For this review, take the finished solid that the model builds, in its own axes (mm). Face numbers are marked on the shaded views. A direction names the side the tool comes from. Give positions to 0.01 mm unless a question says otherwise; leave off trailing zeros. Write each loop counter-clockwise with the first axis right and the second up, starting at its lowest first coordinate (ties: lowest second). Pieces come first, ordered by that corner, then holes. Notation, with made-up numbers: (72.25, 88.25) -> (96.25, 88.25) arc R16 ccw to (96.25, 102.25) -> close; hole circle Ø3 at (17, -26.75). An arc over 180 degrees is marked (long way). Write item = value, one per line.
```python
from build123d import *

# Parameters (mm, degrees)
SKETCH2_W           = 25.4
SKETCH2_H           = 50.8
SKETCH2_W_2         = 19.05
SKETCH2_H_2         = 44.45
BOSS_EXTRUDE1_DEPTH = 127
SKETCH4_R           = 2.38125
CUT_EXTRUDE2_DEPTH  = 25.4


with BuildPart() as part:
    # Sketch2 → Boss-Extrude1 (new body)
    with BuildSketch(Plane(origin=(0, 0, 0), x_dir=(0, 0, -1), z_dir=(1, 0, 0))):
        with Locations((-0.932940239, -1.707357918)):
            Rectangle(SKETCH2_W, SKETCH2_H)
        with Locations((-0.932940239, -1.707357918)):
            Rectangle(SKETCH2_W_2, SKETCH2_H_2, mode=Mode.SUBTRACT)
    extrude(amount=BOSS_EXTRUDE1_DEPTH)

    # Sketch4 → Cut-Extrude2 (cut)
    with BuildSketch(Plane.XY.offset(13.632940239)):
        with Locations((12.7, -8.057357918)):
            Circle(SKETCH4_R)
        with Locations((112.320186583, 10.992642082)):
            Circle(SKETCH4_R)
    extrude(amount=-CUT_EXTRUDE2_DEPTH, mode=Mode.SUBTRACT)


solid = part.part
```
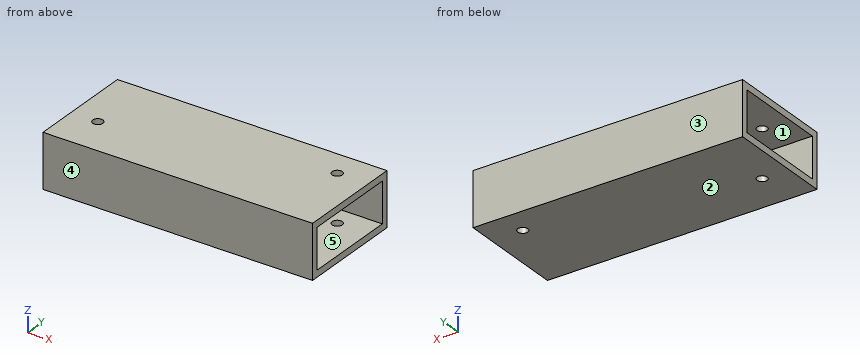
(1) The part is to be moulded in two halves that separate along Y. For the marked faces 1, 2 and 3, say which applies: released by +Y, released by -Y, zero draft, split by the parting line, or undercut.
Answers below:
face_1 = undercut
face_2 = zero draft
face_3 = released by +Y
(2) Take a section at C-C (x = 12.7). Write out the cut boundary in (y, z), plus the area to 3 significant figures.
Answers below:
outline = (-27.11, -11.77) -> (-10.44, -11.77) -> (-10.44, -8.59) -> (-23.93, -8.59) -> (-23.93, 10.46) -> (-10.44, 10.46) -> (-10.44, 13.63) -> (-27.11, 13.63) -> close; (-5.68, -11.77) -> (23.69, -11.77) -> (23.69, 13.63) -> (-5.68, 13.63) -> (-5.68, 10.46) -> (20.52, 10.46) -> (20.52, -8.59) -> (-5.68, -8.59) -> close
area = 413 mm^2
(3) Take a section at A-A (z = 0.5). Write out the cut boundary in (x, y).
Answers below:
outline = (0, -27.11) -> (127, -27.11) -> (127, -23.93) -> (0, -23.93) -> close; (0, 20.52) -> (127, 20.52) -> (127, 23.69) -> (0, 23.69) -> close
(4) Take a section at B-B (x = 33). Write out the cut boundary in (y, z).
Answers below:
outline = (-27.11, -11.77) -> (23.69, -11.77) -> (23.69, 13.63) -> (-27.11, 13.63) -> close; hole (-23.93, -8.59) -> (20.52, -8.59) -> (20.52, 10.46) -> (-23.93, 10.46) -> close
(5) To check wall thickness, follow probe 1 along Z at (x, y) = (121, -11); probe 2 along Y at (x, z) = (77, 1.25); probe 3 along Y at (x, z) = (12.7, -10.85). State the ranges of each line that lie inside material, in increasing order.
Answers below:
probe_1 = -11.77 to -8.59, 10.46 to 13.63
probe_2 = -27.11 to -23.93, 20.52 to 23.69
probe_3 = -27.11 to -10.44, -5.68 to 23.69
(6) Tool access review of the marked faces 4 and 5: name each direction out of +Z, -Z, +X, -X, +Y, -Y from which nothing blocks a thin tool from reaching the whole face with its end or side.
Answers below:
face_4 = +Z, -Z, +X, -X, -Y
face_5 = +X, -X
(7) For pin 1 (6 mm diameter, centred on y = -19, z = -2, fed in from +X), flat-tipped, find the tip position at first contact; note if it passes through.
Answers below:
pin_1 = through
